The model under review builds one solid part; all positions refer to its coordinate system, in mm. A direction names the side the tool comes from. Round coordinates to 2 decimals unless told otherwise and drop trailing zeros. Write each loop counter-clockwise with the first axis right and the second up, starting at its lowest first coordinate (ties: lowest second). Pieces come first, ordered by that corner, then holes. Notation, with made-up numbers: (-22, 82) - (3, 82) arc R3 cw to (3, 86) - close; hole circle Ø6 at (5.5, 12.5). An arc over 180 degrees is marked (long way). Return JSON: item names as keys, results as strings.
from build123d import *

# Parameters (mm, degrees)
F0_W     = 32.0000015199
F0_H     = 32.0000015199
F0_W_2   = 22
F0_H_2   = 22
F1_DEPTH = 12.5
F2_DEPTH = 20


with BuildPart() as f1:
    # F0 (on Top) → F1 (new body)
    with BuildSketch(Plane.XY):
        Rectangle(F0_W, F0_H)
        Rectangle(F0_W_2, F0_H_2, mode=Mode.SUBTRACT)
    extrude(amount=F1_DEPTH)

    # F0 (on Top) → F2 (join)
    with BuildSketch(Plane.XY):
        Rectangle(F0_W, F0_H)
        Rectangle(F0_W_2, F0_H_2, mode=Mode.SUBTRACT)
        Rectangle(F0_W_2, F0_H_2)
    extrude(amount=-F2_DEPTH)


solid = f1.part
(1) Add section A-A (z = 1). Write out the cut boundary in (x, y).
Filled in:
{"outline": "(-16, -16) - (16, -16) - (16, 16) - (-16, 16) - close; hole (-11, -11) - (11, -11) - (11, 11) - (-11, 11) - close"}
(2) Wall thickness on line 1 (Y direction, x = 0, z = 6); line 2 (Z direction, x = -8, y = -10): over which ranges is each line inside the solid? List them lowest first.
Filled in:
{"line 1": "y = -16 to -11, 11 to 16", "line 2": "z = -20 to 0"}
(3) Add section B-B (y = 4.5). Write out the cut boundary in (x, z), plus the area to 3 significant figures.
Filled in:
{"outline": "(-16, -20) - (16, -20) - (16, 12.5) - (11, 12.5) - (11, 0) - (-11, 0) - (-11, 12.5) - (-16, 12.5) - close", "area": "765 mm2"}
(4) Mouldability with a two-part tool opening along X and no side actions: class faces 1 (the flat face through (0, 0, 0)), 2 (the flat face through (-11, 0, 6)), 3 (the flat face through (0, -16, -4)), 4 (the flat face through (-16, 0, -4)) as released by +X, released by -X, zero draft, split by the parting line, or undercut.
Filled in:
{"face 1": "undercut", "face 2": "undercut", "face 3": "zero draft", "face 4": "released by -X"}
(5) Clearance check with a flat-ended pin moving along its axis: pin 1 Ø6.5 at (x, y) = (3, 1.5) entering from +Z. State where the tip first meets the part, or that it passes through.
Filled in:
{"pin 1": "stops at z = 0"}
(6) For faces 5 (the flat face through (0, 16, -4)), 6 (the flat face through (0, 11, 6)), list the 3-axis set-ups (+Z, -Z, +X, -X, +Y, -Y) from which the entire face can be reached by the end or side of a thin tool; tool diameter is ignored.
Filled in:
{"face 5": "+Z, -Z, +X, -X, +Y", "face 6": "+Z"}
